```python
from build123d import *

# Parameters (mm, degrees)
F1_DEPTH  = 12.7
F4_DEPTH  = 3.81
F6_DEPTH  = 8.636
F8_DEPTH  = 25.4
F9_R      = 5.715
F10_DEPTH = 4.318


with BuildPart() as f1:
    # F0 (on Front) → F1 (new body)
    with BuildSketch(Plane.XZ):
        Polygon((-11.43, -5.334), (11.43, -5.334), (11.43, 5.334), (11.43, 16.764), (-11.43, 16.764), (-11.43, 5.334), align=None)
    extrude(amount=F1_DEPTH)

    # F3 (on offset) → F4 (cut)
    with BuildSketch(Plane.XZ.offset(6.35)):
        with BuildLine():
            Line((-9.144, -5.334), (9.144, -5.334))
            Line((9.144, -5.334), (9.144, 5.334))
            ThreePointArc((9.144, 5.334), (0, 14.478), (-9.144, 5.334))
            Line((-9.144, 5.334), (-9.144, -5.334))
        make_face()
    extrude(amount=F4_DEPTH, mode=Mode.SUBTRACT)

    # F5 (on face) → F6 (cut)
    with BuildSketch(Plane.XZ.offset(12.7)):
        with BuildLine():
            Line((6.35, -5.334), (4.846011, 3.81))
            ThreePointArc((4.846011, 3.81), (0, 10.414), (-4.846011, 3.81))
            Line((-4.846011, 3.81), (-6.35, -5.334))
            Line((-6.35, -5.334), (6.35, -5.334))
        make_face()
    extrude(amount=-F6_DEPTH, mode=Mode.SUBTRACT)

    # F7 (on face) → F8 (cut)
    with BuildSketch(Plane.YZ.offset(11.43)):
        Polygon((-2.032, -2.286), (0, -3.302), (0, 14.732), (-2.032, 13.716), align=None)
    extrude(amount=-F8_DEPTH, mode=Mode.SUBTRACT)

    # F9 (on face) → F10 (cut, through all)
    with BuildSketch(Plane(origin=(0, -2.032, 0), x_dir=(-1, 0, 0), z_dir=(0, 1, 0))):
        with Locations((0, 5.334)):
            Circle(F9_R)
    extrude(amount=-F10_DEPTH, mode=Mode.SUBTRACT)


solid = f1.part
```
Geometry: final body of the model. Coordinates: model frame, mm. A direction names the side the tool comes from. Coordinates: 2 decimals unless noted, no trailing zeros. Order: outer loops, then holes, each group sorted by start corner. A loop starts at its lowest first (then second) coordinate and runs counter-clockwise, first axis right, second up. Notation, with made-up numbers: M 0.25,-29.75 L 4.25,-29.75 A25 ccw 4.25,-14.75 Z; hole C 8.5,7.25 d4. An arc over 180 degrees is marked long. Answer in a Markdown table with one row per item. Add a question column.
Q1. Reachability of faces 4 (the flat face through (-9.144, -8, 0)), 5 (the cylindrical face through (0.133, -11.448, 10.412)), 6 (the flat face through (0.2, -2.032, 11.2)), 7 (the flat face through (0, -4.064, -2)), 8 (the flat face through (11.43, -8, 6)) from +Z, -Z, +X, -X, +Y, -Y: full face, straight path, thin tool, end or side. Return the list, or none.
Q2. Section query C-C on z = 3. Return the cut outline in (x, y), and give its area (3 significant figures).
Q3. Line query: L1, parallel to Z at x = 0, y = -3.4; L2, parallel to Y at x = 1.5, z = 11; L3, parallel to Y at x = -5, z = 1.25. Output: solid intervals per line, ascending.
Q4. Mould query, pull axis Z, two halves, no side actions, for faces 1 (the cylindrical face through (0.201, -8.228, 14.476)), 2 (the flat face through (-0.1, -6.35, 11.3)), 3 (the cylindrical face through (-3.072, -4.161, 10.153)). Classes: released by +Z, released by -Z, zero draft, split by the parting line, or undercut.
Q5. Contact query for flat-ended pins moving along their axis: P1, Ø5.5, axis at x = -2, z = 3.5, coming from the -Y side; P2, Ø1.5, axis at x = 6.5, y = -8.5, coming from the -Z side; P3, Ø3, axis at x = 1, y = -9, coming from the -Z side; P4, Ø13, axis at x = 5, z = 5, coming from the +Y side. Output: stop coordinate, or through.
Q6. Section query A-A on x = -1. Return the cut outline in (y, z).
Q7. Section query D-D on y = -2.5. Return the cut outline in (x, z) (3 decimals).
Q8. Section query B-B on y = -7. Return the cut outline in (x, z).
Completed:
| question | item | result |
|---|---|---|
| 1 | face 4 | -Z |
| 1 | face 5 | +Y, -Y |
| 1 | face 6 | +X, -X, +Y |
| 1 | face 7 | -Z, -Y |
| 1 | face 8 | +Z, -Z, +X, +Y, -Y |
| 2 | outline | M -11.43,-12.7 L -4.98,-12.7 L -4.98,-10.16 L -9.14,-10.16 L -9.14,-6.35 L -5.22,-6.35 L -5.22,-2.03 L -11.43,-2.03 Z; M 4.98,-12.7 L 11.43,-12.7 L 11.43,-2.03 L 5.22,-2.03 L 5.22,-6.35 L 9.14,-6.35 L 9.14,-10.16 L 4.98,-10.16 Z |
| 2 | area | 104 mm2 |
| 3 | L1 | z = -5.33 to -0.38, 11.05 to 16.76 |
| 3 | L2 | y = -12.7 to -10.16, -6.35 to -2.03 |
| 3 | L3 | y = -4.06 to -2.03 |
| 4 | face 1 | released by -Z |
| 4 | face 2 | zero draft |
| 4 | face 3 | undercut |
| 5 | P1 | passes through |
| 5 | P2 | stops at z = 10.91 |
| 5 | P3 | stops at z = 10.02 |
| 5 | P4 | stops at y = -2.03 |
| 6 | outline | M -12.7,10.31 L -10.16,10.31 L -10.16,14.42 L -6.35,14.42 L -6.35,10.96 L -2.03,10.96 L -2.03,13.72 L 0,14.73 L 0,16.76 L -12.7,16.76 Z; M -4.06,-5.33 L 0,-5.33 L 0,-3.3 L -2.03,-2.29 L -2.03,-0.29 L -4.06,-0.29 Z |
| 7 | outline | M -11.43,-5.334 L 11.43,-5.334 L 11.43,16.764 L -11.43,16.764 Z; hole C 0,5.334 d11.43 |
| 8 | outline | M -11.43,-5.33 L -9.14,-5.33 L -9.14,5.33 A9.14 cw 9.14,5.33 L 9.14,-5.33 L 11.43,-5.33 L 11.43,16.76 L -11.43,16.76 Z |
